For this review, use the dimensioned drawing (mm, ordinates from the lowest corner) and the shaded views. Coordinates: 2 decimals unless noted, no trailing zeros. Write each loop counter-clockwise with the first axis right and the second up, starting at its lowest first coordinate (ties: lowest second). Pieces come first, ordered by that corner, then holes. Notation, with made-up numbers: M 1.25,54 L 21.25,54 A19 ccw 21.25,73 Z; hole C -29,-22.75 d11. An arc over 180 degrees is marked long. Return JSON: item names as keys, results as strings.
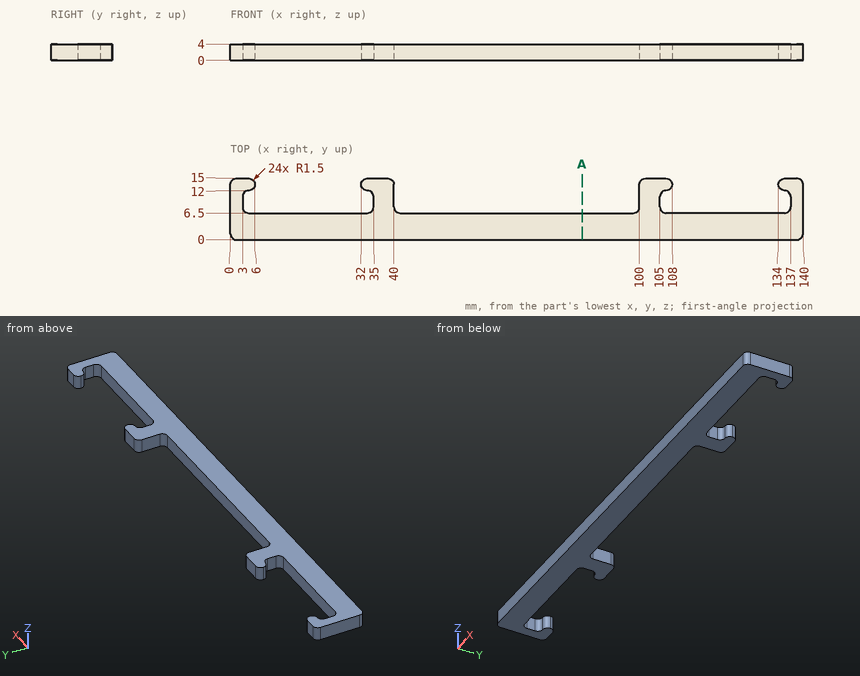
1. Wall thickness on L1, parallel to X at y = 10.5, z = 2.95; L2, parallel to X at y = 7, z = 1.9; L3, parallel to Y at x = 21, z = 0.9: over which ranges is each line inside the solid? List them lowest first. Write a range as from..to.
Checks:
{"L1": "0..3, 35..40, 100..105, 137..140", "L2": "0..3.38, 34.62..40.38, 99.62..105.38, 136.62..140", "L3": "0..6.5"}
2. We need section A-A (x = 86). State the section outline as (y, z) points.
Checks:
{"outline": "M 0,0 L 6.5,0 L 6.5,4 L 0,4 Z"}
3. Clearance check with a flat-ended pin moving along its axis: pin 1 Ø1.2 at (x, z) = (120.5, 2) entering from +Y. State where the tip first meets the part, or that it passes through.
Checks:
{"pin 1": "y = 6.5"}
